Design review of the part shown in the three views and the two pictorial views. Dimensions are in mm from the part's minimum x, y and z. Give positions to 0.01 mm unless a question says otherwise; leave off trailing zeros. Loops run counter-clockwise (first coordinate to the right, second up) from the corner with the lowest first, then second, coordinate; pieces in that order, holes last. Notation, with made-up numbers: (-33.75, 31) -> (-5.75, 31) arc R25 ccw to (-5.75, 57) -> close; hole circle Ø2 at (-6, -37). An arc over 180 degrees is marked (long way). Answer as CSV lines item,"result". Start each with the question number.
Item 1: Add section D-D on y = 26. State the section outline as (x, z) points, plus the area to 3 significant figures.
Item 2: Add section C-C on z = 39.5. State the section outline as (x, y) points, plus the area to 3 significant figures.
Item 3: Add section A-A on z = 23. State the section outline as (x, y) points, plus the area to 3 significant figures.
Item 4: For L1, parallel to X at y = 46, z = 25; L2, parallel to Z at x = 31.5, y = 122.5; L3, parallel to Z at x = 20, y = 75, list the stretches that pass through material, from the lowest coordinate up. Write a range as from..to.
Item 5: The part is to be moulded in two halves that separate along Z. For the marked faces 1 and 2, say which applies: +Z half, -Z half, draft (parallel to the pull), parting line (faces both ways), or undercut.
Item 6: Clearance check with flat-ended pins moving along their axes: P1, Ø1, axis at x = 24, y = 120, coming from the -Z side; P2, Ø3, axis at y = 123.5, z = 7, coming from the -X side; P3, Ø10, axis at x = 40, y = 101.5, coming from the -Z side; P4, Ø23, axis at x = 15.5, z = 24, coming from the +Y side. State where each tip first meets the part, or that it passes through.
Item 7: Add section B-B on x = 7. State the section outline as (y, z) points, plus the area to 3 significant figures.
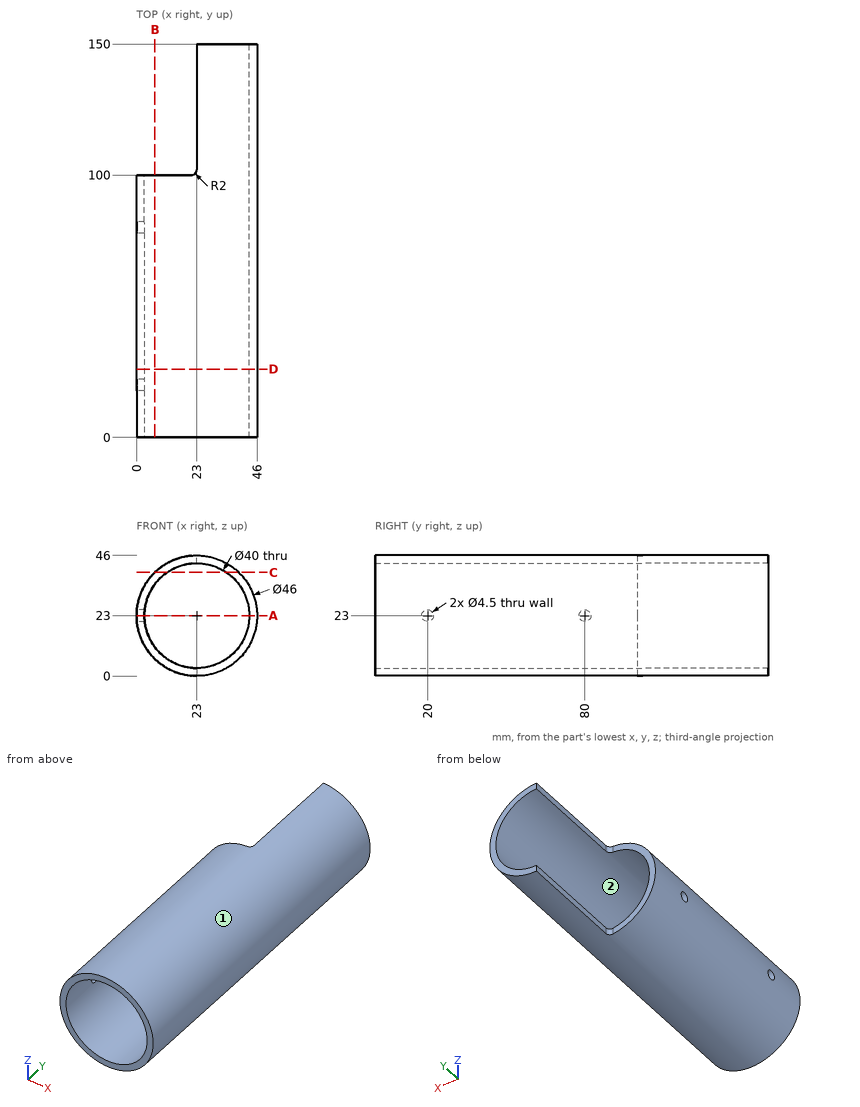
Computed values:
1,outline,"circle Ø46 at (23, 23); hole circle Ø40 at (23, 23)"
1,area,"405 mm²"
2,outline,"(6.98, 0) -> (11.7, 0) -> (11.7, 100) -> (6.98, 100) -> close; (34.3, 0) -> (39.02, 0) -> (39.02, 150) -> (34.3, 150) -> close"
2,area,"1,180 mm²"
3,outline,"(0, 0) -> (3, 0) -> (3, 17.75) -> (0, 17.75) -> close; (0, 22.25) -> (3, 22.25) -> (3, 77.75) -> (0, 77.75) -> close; (0, 82.25) -> (3, 82.25) -> (3, 100) -> (0, 100) -> close; (43, 0) -> (46, 0) -> (46, 150) -> (43, 150) -> close"
3,area,"723 mm²"
4,L1,"0.09..3.1, 42.9..45.91"
4,L2,"1.63..4.9, 41.1..44.37"
4,L3,"0.2..3.23, 42.77..45.8"
5,face 1,"parting line"
5,face 2,"undercut"
6,P1,"z = 0.01"
6,P2,"x = 32.68"
6,P3,"z = 3.38"
6,P4,"through"
7,outline,"(0, 6.48) -> (100, 6.48) -> (100, 11) -> (0, 11) -> close; (0, 35) -> (100, 35) -> (100, 39.52) -> (0, 39.52) -> close"
7,area,"905 mm²"
